Here's the drawing with two shaded views (mm, measured from the low corner). I have some questions. A direction names the side the tool comes from. Coordinates: 2 decimals unless noted, no trailing zeros. Write each loop counter-clockwise with the first axis right and the second up, starting at its lowest first coordinate (ties: lowest second). Pieces come first, ordered by that corner, then holes.
Item 1: If we section it at B-B (x = 34): Please give me the cut outline in (y, z), then the cut area to 3 significant figures.
Item 2: I'm going to push flat-ended pins straight in: pin 1 Ø3 at (x, z) = (22.5, 18) entering from +Y; pin 2 Ø4 at (x, y) = (28.5, 8) entering from -Z; pin 3 Ø2 at (x, z) = (5, 5.5) entering from +Y. Where does each tip first touch, or does it pass through?
Item 3: We'd pull the mould along X, two halves only. Please class the marked faces 4, 5 and 6: +X half, -X half, draft (parallel to the pull), parting line (faces both ways), or undercut.
Item 4: If we section it at A-A (x = 7.5): Please give me the cut outline in (y, z) (1 decimal).
Item 5: If I drill on line 1 (X direction, y = 11, z = 3.25); line 2 (Y direction, x = 24, z = 11.75); line 3 (Y direction, x = 32, z = 16) (1 decimal), over which ranges is the centre line in solid material (lowest first)?
Item 6: For the marked faces 1, 2 and 3, which set-ups out of +Z, -Z, +X, -X, +Y, -Y let a thin tool reach every point of the face, with its end or its side?
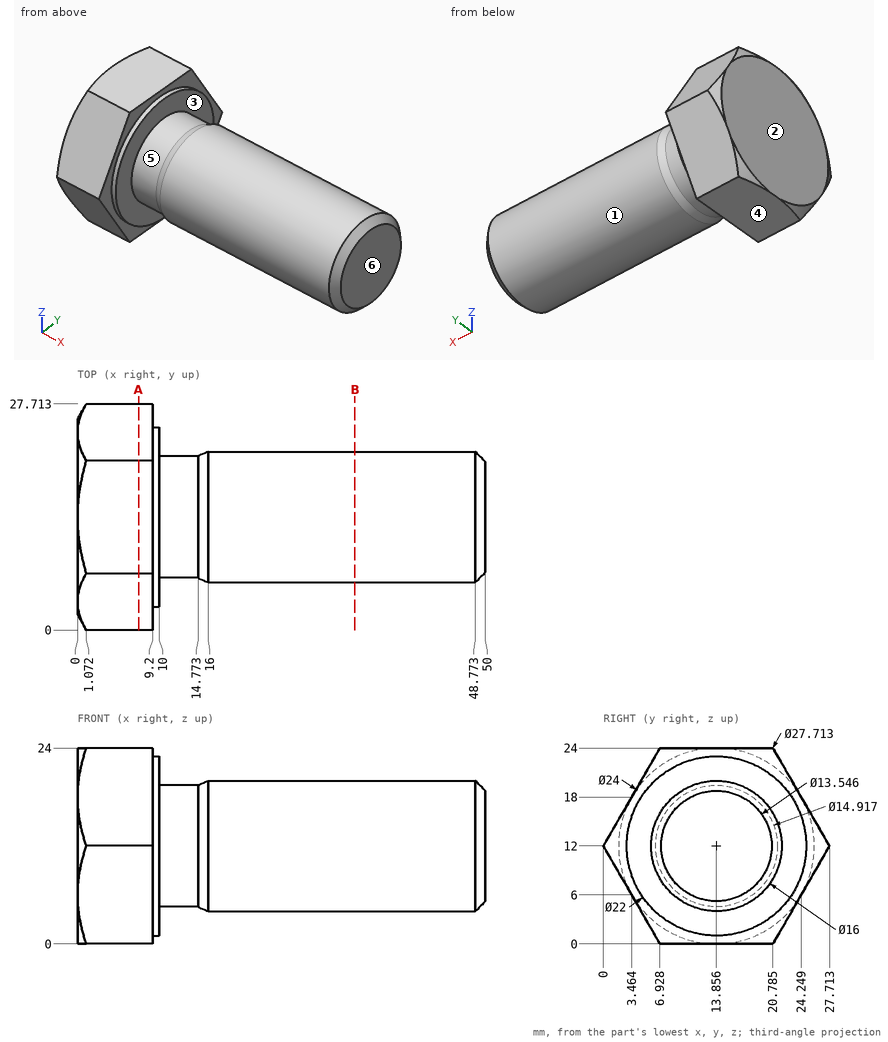
Answer list:
1. outline: circle Ø16 at (13.86, 12)
1. area: 201 mm2
2. pin 1: stops at y = 20.47
2. pin 2: stops at z = 4.99
2. pin 3: stops at y = 24.54
3. face 4: draft
3. face 5: undercut
3. face 6: +X half
4. outline: (0, 12) - (6.9, 0) - (20.8, 0) - (27.7, 12) - (20.8, 24) - (6.9, 24) - close
5. line 1: x = 0 to 10
5. line 2: y = 5.86 to 21.85
5. line 3: y = 6.9 to 20.8
6. face 1: +X
6. face 2: +Z, -Z, -X, +Y, -Y
6. face 3: none
